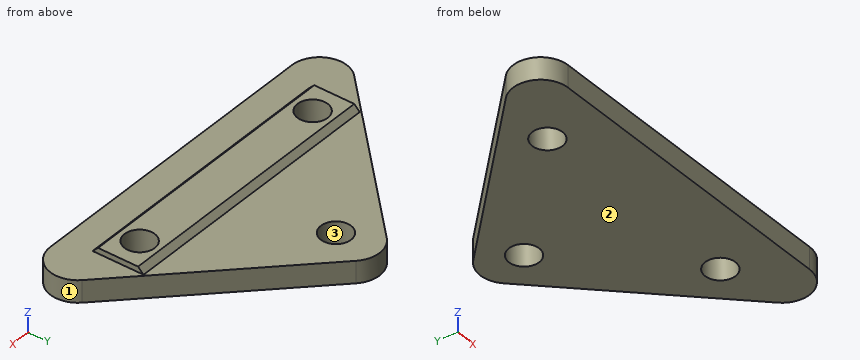
from build123d import *

# Parameters (mm, degrees)
F1_DEPTH      = 4
F3_DEPTH      = 25
F3_DEPTH_BACK = 25
F4_D          = 5.5


with BuildPart() as f1:
    # F0 (on Top) → F1 (new body)
    with BuildSketch(Plane.XY):
        with BuildLine():
            ThreePointArc((3.5355339059, 36.4644660941), (0, 37.9289321881), (-3.5355339059, 36.4644660941))
            Line((-3.5355339059, 36.4644660941), (-31.4644660941, 8.5355339059))
            ThreePointArc((-31.4644660941, 8.5355339059), (-32.5483298507, 3.0865828382), (-27.9289321881, 0))
            Line((-27.9289321881, 0), (27.9289321881, 0))
            ThreePointArc((27.9289321881, 0), (32.5483298507, 3.0865828382), (31.4644660941, 8.5355339059))
            Line((31.4644660941, 8.5355339059), (3.5355339059, 36.4644660941))
        make_face()
    extrude(amount=F1_DEPTH)

    # F2 (on Right) → F3 (join, two sides)
    with BuildSketch(Plane.YZ) as f3_sk:
        Polygon((5.36, 4), (14.64, 4), (13.64, 5), (6.36, 5), align=None)
    extrude(amount=F3_DEPTH)
    extrude(f3_sk.sketch, amount=-F3_DEPTH_BACK)

    # F4 (through all)
    with Locations(Plane(origin=(0, 0, 0), x_dir=(1, 0, 0), z_dir=(0, 0, -1))):
        with Locations((-20, -10), (0, -30), (20, -10)):
            Hole(F4_D / 2)


solid = f1.part
Work out the finished part from the listing and answer in its coordinate system (mm). Face numbers are marked on the shaded views. Coordinates: 2 decimals unless noted, no trailing zeros. Loops run counter-clockwise (first coordinate to the right, second up) from the corner with the lowest first, then second, coordinate; pieces in that order, holes last. Notation, with made-up numbers: M -29.75,-33 L 6.25,-33 A29 ccw 6.25,-8 Z; hole C 33.25,9.5 d9. An arc over 180 degrees is marked long. Answer in a Markdown table with one row per item. Add a question column.
1. The mould has two halves that part along X. Classify the marked faces 1, 2 and 3: pulls with the +X half, pulls with the -X half, needs draft (parallel to the pull), parting line crosses it, or undercut.
2. Find section C-C, the plane z = 1.1. Write down the section's boundary in (x, y).
3. Flat-ended cylindrical pins translate along their axes: P1, Ø0.5, axis at y = 11, z = 4.5, coming from the +X side; P2, Ø8, axis at x = -26, y = 9.5, coming from the -Z side; P3, Ø4.5, axis at x = 20, y = 10, coming from the -Z side; P4, Ø7, axis at x = 0, y = 30, coming from the +Z side. Find the tip coordinate at first contact, or state that the pin passes through.
4. Find section B-B, the plane y = 30. Write down the section's boundary in (x, z).
5. Find section D-D, the plane y = 10. Write down the section's boundary in (x, z).
6. Find section A-A, the plane x = 0. Write down the section's boundary in (y, z).
7. Consider L1, parallel to X at y = 8, z = 4.05; L2, parallel to Z at x = -7.5, y = 16; L3, parallel to X at y = 7.5, z = 1.95. Determine where each line is inside the solid, lowest interval first.
Reported:
| question | item | result |
|---|---|---|
| 1 | face 1 | pulls with the +X half |
| 1 | face 2 | needs draft |
| 1 | face 3 | undercut |
| 2 | outline | M -31.46,8.54 A5 ccw -27.93,0 L 27.93,0 A5 ccw 31.46,8.54 L 3.54,36.46 A5 ccw -3.54,36.46 Z; hole C -20,10 d5.5; hole C 0,30 d5.5; hole C 20,10 d5.5 |
| 3 | P1 | stops at x = 25 |
| 3 | P2 | stops at z = 0 |
| 3 | P3 | passes through |
| 3 | P4 | stops at z = 4 |
| 4 | outline | M -10,0 L -2.75,0 L -2.75,4 L -10,4 Z; M 2.75,0 L 10,0 L 10,4 L 2.75,4 Z |
| 5 | outline | M -30,0 L -22.75,0 L -22.75,5 L -25,5 L -25,4 L -30,4 Z; M -17.25,0 L 17.25,0 L 17.25,5 L -17.25,5 Z; M 22.75,0 L 30,0 L 30,4 L 25,4 L 25,5 L 22.75,5 Z |
| 6 | outline | M 0,0 L 27.25,0 L 27.25,4 L 14.64,4 L 13.64,5 L 6.36,5 L 5.36,4 L 0,4 Z; M 32.75,0 L 37.93,0 L 37.93,4 L 32.75,4 Z |
| 7 | L1 | x = -25 to -21.89, -18.11 to 18.11, 21.89 to 25 |
| 7 | L2 | z = 0 to 4 |
| 7 | L3 | x = -32.26 to -21.15, -18.85 to 18.85, 21.15 to 32.26 |
